from build123d import *

# Parameters (mm, degrees)
SKETCH1_R           = 9
SKETCH1_R_2         = 5.5
BOSS_EXTRUDE1_DEPTH = 5
SKETCH2_R           = 9
BOSS_EXTRUDE2_DEPTH = 3
BOSS_EXTRUDE3_DEPTH = 4
SKETCH4_OUTSIDE_W   = 26.244
SKETCH4_OUTSIDE_H   = 26.244
SKETCH4_OUTSIDE_R   = 9
CUT_EXTRUDE1_DEPTH  = 17.235607036


with BuildPart() as part:
    # Sketch1 → Boss-Extrude1 (new body)
    with BuildSketch(Plane.XY):
        Circle(SKETCH1_R)
        Circle(SKETCH1_R_2, mode=Mode.SUBTRACT)
    extrude(amount=BOSS_EXTRUDE1_DEPTH)

    # Sketch2 → Boss-Extrude2 (add)
    with BuildSketch(Plane.XY.offset(5)):
        Circle(SKETCH2_R)
    extrude(amount=BOSS_EXTRUDE2_DEPTH)

    # Sketch3 → Boss-Extrude3 (add, symmetric)
    with BuildSketch(Plane(origin=(0, 0, 0), x_dir=(1, 0, 0), z_dir=(0, 1, 0))):
        Polygon((-5.333731513, -11), (-5.333731513, -8), (-9, -8), (-9, -13.502081056), (-1.07179677, -18.079431325), (1.07179677, -18.079431325), (9, -13.502081056), (9, -8), (5.333731513, -8), (5.333731513, -11), (0, -14.079431325), align=None)
    extrude(amount=BOSS_EXTRUDE3_DEPTH, both=True)

    # Sketch4 outside → Cut-Extrude1 (cut, through all)
    with BuildSketch(Plane.XY.offset(8)):
        Rectangle(SKETCH4_OUTSIDE_W, SKETCH4_OUTSIDE_H)
        with Locations(Location((0, 0, 0), (0, 0, 206.387799961))):
            Circle(SKETCH4_OUTSIDE_R, mode=Mode.SUBTRACT)
    extrude(amount=CUT_EXTRUDE1_DEPTH, mode=Mode.SUBTRACT)


solid = part.part
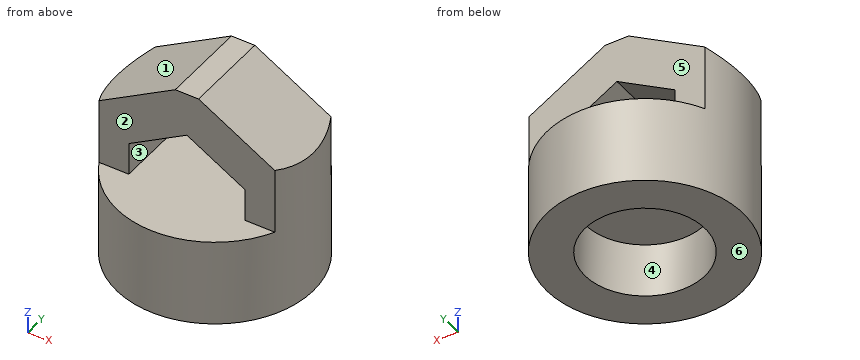
Source: CAD feature listing. Evaluate the final solid. Frame: model axes, mm. Face numbers are marked on the shaded views. A direction names the side the tool comes from. Round coordinates to 2 decimals unless told otherwise and drop trailing zeros. Loops run counter-clockwise (first coordinate to the right, second up) from the corner with the lowest first, then second, coordinate; pieces in that order, holes last. Notation, with made-up numbers: M 22,65.25 L 26,65.25 A36 ccw 26,101.25 Z; hole C -36.5,20.5 d2. An arc over 180 degrees is marked long. Return JSON: item names as keys, results as strings. Group by question number.
1. Section query A-A on y = 0. Output: boundary loops of the cut face in (x, z), and give its area (3 significant figures).
2. Section query C-C on z = 5.5. Output: boundary loops of the cut face in (x, y), and give its area (3 significant figures).
3. Reachability of the marked faces 4, 5 and 6 from +Z, -Z, +X, -X, +Y, -Y: full face, straight path, thin tool, end or side. Return the list, or none.
4. Material intervals for line 1 along Y through (x, z) = (0, 1.25); line 2 along Z through (x, y) = (-6, 6.25); line 3 along Z through (x, y) = (-2.5, -2.25), sorted ascending. Write a range as from..to.
5. Pin query (flat end, axial travel): pin 1 (3 mm diameter, centred on x = 2.5, z = 14, fed in from -Y); pin 2 (3.5 mm diameter, centred on x = -1, y = 2, fed in from -Z); pin 3 (1 mm diameter, centred on y = 4, z = 4.5, fed in from +X). Return the tip coordinate at first contact, or that it passes through.
6. Mould query, pull axis X, two halves, no side actions, for the marked faces 1, 2 and 3. Classes: released by +X, released by -X, zero draft, split by the parting line, or undercut.
7. Section query B-B on z = 3.5. Output: boundary loops of the cut face in (x, y), and give its area (3 significant figures).
Checks:
{
 "1": {"outline": "M -9,0 L -5.5,0 L -5.5,5 L 5.5,5 L 5.5,0 L 9,0 L 9,13.5 L 1.07,18.08 L -1.07,18.08 L -9,13.5 Z; hole M -5.33,8 L 5.33,8 L 5.33,11 L 0,14.08 L -5.33,11 Z", "area": "186 mm²"},
 "2": {"outline": "C 0,0 d18", "area": "254 mm²"},
 "3": {"face 4": "-Z", "face 5": "+Z, +X, -X, +Y", "face 6": "-Z, +X, -X, +Y, -Y"},
 "4": {"line 1": "y = -9..-5.5, 5.5..9", "line 2": "z = 0..8", "line 3": "z = 5..8, 12.64..17.25"},
 "5": {"pin 1": "stops at y = -4", "pin 2": "stops at z = 5", "pin 3": "stops at x = 8.29"},
 "6": {"face 1": "released by -X", "face 2": "zero draft", "face 3": "undercut"},
 "7": {"outline": "C 0,0 d18; hole C 0,0 d11", "area": "159 mm²"}
}
